Can you work these out from the model? Positions are in its coordinate system, mm. A direction names the side the tool comes from. Coordinates: 2 decimals unless noted, no trailing zeros. Order: outer loops, then holes, each group sorted by start corner. A loop starts at its lowest first (then second) coordinate and runs counter-clockwise, first axis right, second up. Notation, with made-up numbers: (30.5, -21.75) -> (39.5, -21.75) arc R26 ccw to (39.5, -6.75) -> close; hole circle Ø7 at (33, 80.5). An arc over 180 degrees is marked (long way). Use a Markdown table: item, result. Add a question column.
1. Suppose I cut it at B-B, the plane y = 0. List the corners of the cut face in (x, z) for me, then the cut area to 3 significant figures.
2. If I drill on line 1 along Y through (x, z) = (0, 3.7); line 2 along Z through (x, y) = (6.75, 6.25), over which ranges is the centre line in solid material (lowest first)? Write a range as from..to.
3. For pin 1 Ø12 at (x, y) = (1, -6) entering from +Z; pin 2 Ø0.5 at (x, z) = (-9, 5.5) entering from -Y; pin 3 Ø1 at (y, z) = (0, 6) entering from +X, each with a flat end and sliding along its axis, tell me the tip position at first contact or that it passes through.
4. Suppose I cut it at D-D, the plane y = 4.75. List the corners of the cut face in (x, z) for me, then the cut area to 3 significant figures.
5. Suppose I cut it at A-A, the plane x = 0. List the corners of the cut face in (y, z) for me.
6. For faces 1 (the cylindrical face through (-2.17, -9.76, 2.46)), 2 (the flat face through (-9.3, 0, 6)), 3 (the flat face through (8.7, 0, 6)), 4 (the flat face through (9.3, 0, 6)), which set-ups out of +Z, -Z, +X, -X, +Y, -Y let a thin tool reach every point of the face, with its end or its side?
7. Suppose I cut it at C-C, the plane z = 2.5. List the corners of the cut face in (x, y) for me.
```python
from build123d import *

# Parameters (mm, degrees)
F0_W     = 0.6
F0_H     = 1.8
F1_DEPTH = 6.3
F0_R     = 10
F0_R_2   = 8
F2_DEPTH = 5


with BuildPart() as f1:
    # F0 (on Top) → F1 (new body)
    with BuildSketch(Plane.XY):
        with Locations((-9, 0)):
            Rectangle(F0_W, F0_H)
    extrude(amount=F1_DEPTH)



with BuildPart() as f1b:
    # F0 (on Top) → F1, piece 2 (new body)
    with BuildSketch(Plane.XY):
        with Locations((9, 0)):
            Rectangle(F0_W, F0_H)
    extrude(amount=F1_DEPTH)


with BuildPart() as f1_1:
    add(f1.part)

    add(f1b.part)  # F2 merges F1b
    # F0 (on Top) → F2 (join)
    with BuildSketch(Plane.XY):
        Circle(F0_R)
        with Locations((-9, 0)):
            Rectangle(F0_W, F0_H, mode=Mode.SUBTRACT)
        Circle(F0_R_2, mode=Mode.SUBTRACT)
        with Locations((9, 0)):
            Rectangle(F0_W, F0_H, mode=Mode.SUBTRACT)
    extrude(amount=F2_DEPTH)


solid = f1_1.part
```
Worked out:
| question | item | result |
|---|---|---|
| 1 | outline | (-10, 0) -> (-8, 0) -> (-8, 5) -> (-8.7, 5) -> (-8.7, 6.3) -> (-9.3, 6.3) -> (-9.3, 5) -> (-10, 5) -> close; (8, 0) -> (10, 0) -> (10, 5) -> (9.3, 5) -> (9.3, 6.3) -> (8.7, 6.3) -> (8.7, 5) -> (8, 5) -> close |
| 1 | area | 21.6 mm² |
| 2 | line 1 | y = -10..-8, 8..10 |
| 2 | line 2 | z = 0..5 |
| 3 | pin 1 | stops at z = 5 |
| 3 | pin 2 | stops at y = -0.9 |
| 3 | pin 3 | stops at x = 9.3 |
| 4 | outline | (-8.8, 0) -> (-6.44, 0) -> (-6.44, 5) -> (-8.8, 5) -> close; (6.44, 0) -> (8.8, 0) -> (8.8, 5) -> (6.44, 5) -> close |
| 4 | area | 23.6 mm² |
| 5 | outline | (-10, 0) -> (-8, 0) -> (-8, 5) -> (-10, 5) -> close; (8, 0) -> (10, 0) -> (10, 5) -> (8, 5) -> close |
| 6 | face 1 | +Z, -Z |
| 6 | face 2 | +Z, -X, +Y, -Y |
| 6 | face 3 | +Z, +Y, -Y |
| 6 | face 4 | +Z, +X, +Y, -Y |
| 7 | outline | circle Ø20 at (0, 0); hole circle Ø16 at (0, 0) |
